from build123d import *

# Parameters (mm, degrees)
F0_R          = 1.5
F1_DEPTH      = 1.5
F1_DEPTH_BACK = 1.5
F2_R          = 0.5


with BuildPart() as f1:
    # F0 (on Front) → F1 (new body, two sides)
    with BuildSketch(Plane.XZ) as f1_sk:
        with BuildLine():
            Line((-20, 0), (20, 0))
            ThreePointArc((20, 0), (0, 20), (-20, 0))
        make_face()
        with Locations((0, 5)):
            Circle(F0_R, mode=Mode.SUBTRACT)
    extrude(amount=F1_DEPTH)
    extrude(f1_sk.sketch, amount=-F1_DEPTH_BACK)

    # F2
    f2_edges = [f1.edges().sort_by_distance(p)[0] for p in [
        (0, -1.5, 20),
        (0, 1.5, 20),
    ]]
    fillet(f2_edges, radius=F2_R)


solid = f1.part
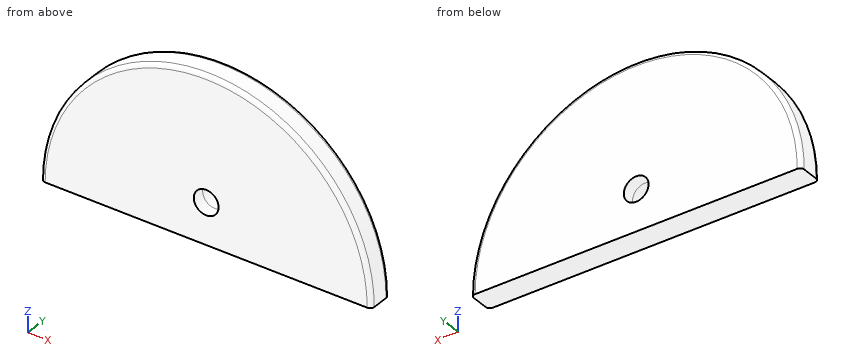
Geometry check sheet. Reference: the model listing, model coordinates, mm. Give positions to 0.01 mm unless a question says otherwise; leave off trailing zeros. Order: outer loops, then holes, each group sorted by start corner. A loop starts at its lowest first (then second) coordinate and runs counter-clockwise, first axis right, second up. Notation, with made-up numbers: (55, -38.5) - (97, -38.5) arc R18 ccw to (97, -11.5) - close; hole circle Ø6 at (49, -33.5). An arc over 180 degrees is marked (long way). Answer as a JSON object with one key per item and string values.
(1) Cross-section at B-B (y = -0.4). Record the cut outline in (x, z).
Report:
{"outline": "(-20, 0) - (20, 0) arc R20 ccw to start; hole circle Ø3 at (0, 5)"}
(2) Depth check by flat-ended pin: pin 1 Ø1.5 at (y, z) = (1, 17) entering from -X; pin 2 Ø2.5 at (x, z) = (0, 5) entering from +Y; pin 3 Ø1 at (y, z) = (0, 11.5) entering from -X. Enter the tip coordinate at first touch or a pass-through.
Report:
{"pin 1": "x = -11.66", "pin 2": "through", "pin 3": "x = -16.7"}
(3) Cross-section at A-A (x = 0). Record the cut outline in (y, z), then the cut area to 3 significant figures.
Report:
{"outline": "(-1.5, 0) - (1.5, 0) - (1.5, 3.5) - (-1.5, 3.5) - close; (-1.5, 6.5) - (1.5, 6.5) - (1.5, 19.5) arc R0.5 ccw to (1, 20) - (-1, 20) arc R0.5 ccw to (-1.5, 19.5) - close", "area": "50.9 mm^2"}
(4) Material ranges on line 1 (Z direction, x = 0, y = 0.6); line 2 (X direction, y = 1, z = 8); line 3 (Z direction, x = -5, y = 0.85), recorded low to high.
Report:
{"line 1": "0 to 3.5, 6.5 to 20", "line 2": "-18.33 to 18.33", "line 3": "0 to 19.36"}
